Could you check a few things on this model? Use its own coordinates, in mm. Give positions to 0.01 mm unless a question says otherwise; leave off trailing zeros. Write each loop counter-clockwise with the first axis right and the second up, starting at its lowest first coordinate (ties: lowest second). Pieces come first, ordered by that corner, then holes. Notation, with made-up numbers: (12, 75) -> (28, 75) arc R16 ccw to (28, 79) -> close; hole circle Ø5 at (84.5, -14). An arc over 180 degrees is marked (long way). One line per question, with ' | ' between items.
from build123d import *

# Parameters (mm, degrees)
F0_W     = 35
F0_H     = 150
F0_R     = 5.5
F1_DEPTH = 2.5


with BuildPart() as f1:
    # F0 (on Front) → F1 (new body, symmetric)
    with BuildSketch(Plane.XZ):
        Rectangle(F0_W, F0_H)
        with Locations((0, -50)):
            Circle(F0_R, mode=Mode.SUBTRACT)
        Circle(F0_R, mode=Mode.SUBTRACT)
    extrude(amount=F1_DEPTH, both=True)


solid = f1.part
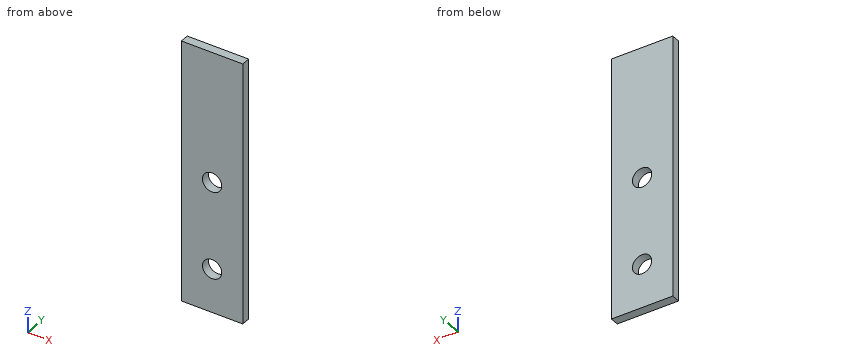
Q1. Imagine slicing it at C-C on y = -0.55. Please give me the cut outline in (x, z).
Answer below:
outline: (-17.5, -75) -> (17.5, -75) -> (17.5, 75) -> (-17.5, 75) -> close; hole circle Ø11 at (0, -50); hole circle Ø11 at (0, 0)
Q2. Imagine slicing it at A-A on x = 0. Please give me the cut outline in (y, z).
Answer below:
outline: (-2.5, -75) -> (2.5, -75) -> (2.5, -55.5) -> (-2.5, -55.5) -> close; (-2.5, -44.5) -> (2.5, -44.5) -> (2.5, -5.5) -> (-2.5, -5.5) -> close; (-2.5, 5.5) -> (2.5, 5.5) -> (2.5, 75) -> (-2.5, 75) -> close
Q3. Will this pin go through, and if not, where does the flat tip stop? pin 1 (6.5 mm diameter, centred on x = 0, z = 0, fed in from +Y).
Answer below:
pin 1: passes through
Q4. Imagine slicing it at B-B on z = -50. Please give me the cut outline in (x, y).
Answer below:
outline: (-17.5, -2.5) -> (-5.5, -2.5) -> (-5.5, 2.5) -> (-17.5, 2.5) -> close; (5.5, -2.5) -> (17.5, -2.5) -> (17.5, 2.5) -> (5.5, 2.5) -> close
Q5. If I drill on line 1 along Z through (x, y) = (0, 1.1); line 2 along Z through (x, y) = (-1, -0.35); line 3 along X through (y, z) = (-1.95, -54.5), over which ranges is the centre line in solid material (lowest first)?
Answer below:
line 1: z = -75 to -55.5, -44.5 to -5.5, 5.5 to 75 | line 2: z = -75 to -55.41, -44.59 to -5.41, 5.41 to 75 | line 3: x = -17.5 to -3.16, 3.16 to 17.5
